from build123d import *

# Parameters (mm, degrees)
SKETCH1_W           = 30
SKETCH1_H           = 38
BOSS_EXTRUDE1_DEPTH = 2
SKETCH2_R           = 0.5
BOSS_EXTRUDE2_DEPTH = 0.8
SKETCH5_W           = 1
SKETCH5_H           = 38
BOSS_EXTRUDE4_DEPTH = 1
SKETCH6_W           = 1
SKETCH6_H           = 38
BOSS_EXTRUDE5_DEPTH = 20
SKETCH8_W           = 18
SKETCH8_H           = 38
BOSS_EXTRUDE6_DEPTH = 3.5
CUT_EXTRUDE1_DEPTH  = 29
SKETCH12_W          = 80
SKETCH12_H          = 38
BOSS_EXTRUDE7_DEPTH = 1


with BuildPart() as part:
    # Sketch1 → Boss-Extrude1 (new body)
    with BuildSketch(Plane.XY):
        Rectangle(SKETCH1_W, SKETCH1_H)
    extrude(amount=BOSS_EXTRUDE1_DEPTH)

    # Sketch2 → Boss-Extrude2 (add)
    with BuildSketch(Plane(origin=(0, 0, 0), x_dir=(-1, 0, 0), z_dir=(0, 0, -1))):
        with Locations(Location((14, 16.5, 0), (0, 0, 180))):
            Circle(SKETCH2_R)
        with Locations(Location((14, -17.5, 0), (0, 0, 180))):
            Circle(SKETCH2_R)
    extrude(amount=BOSS_EXTRUDE2_DEPTH)

    # Sketch5 → Boss-Extrude4 (add)
    with BuildSketch(Plane.XY.offset(2)):
        with Locations((14.5, 0)):
            Rectangle(SKETCH5_W, SKETCH5_H)
    extrude(amount=BOSS_EXTRUDE4_DEPTH)

    # Sketch6 → Boss-Extrude5 (add)
    with BuildSketch(Plane(origin=(15, 0, 0), x_dir=(0, 0, -1), z_dir=(1, 0, 0))):
        with Locations((-2.5, 0)):
            Rectangle(SKETCH6_W, SKETCH6_H)
    extrude(amount=BOSS_EXTRUDE5_DEPTH)

    # Mirror2: part across plane


with BuildPart() as part_1:
    add(part.part)
    add(part.part.mirror(Plane(origin=(25, 0, 0), x_dir=(0, 0, 1), z_dir=(1, 0, 0))))

    # Sketch8 → Boss-Extrude6 (add)
    with BuildSketch(Plane.XY.offset(3)):
        with Locations((25, 0)):
            Rectangle(SKETCH8_W, SKETCH8_H)
    extrude(amount=BOSS_EXTRUDE6_DEPTH)

    # Sketch9 → Cut-Extrude1 (cut)
    with BuildSketch(Plane.ZY.offset(15)):
        Polygon((2, -0.8), (2, 0.8), (1.5, 0.8), (1.5, 1.2), (0.5, 1.2), (0.5, -1.2), (1.5, -1.2), (1.5, -0.8), align=None)
    cut_extrude1 = extrude(amount=-CUT_EXTRUDE1_DEPTH, mode=Mode.SUBTRACT)

    # Mirror3: Cut-Extrude1 across plane
    add(cut_extrude1.mirror(Plane(origin=(25, 0, 0), x_dir=(0, 0, 1), z_dir=(1, 0, 0))), mode=Mode.SUBTRACT)

    # Sketch12 → Boss-Extrude7 (add)
    with BuildSketch(Plane.XY.offset(6.5)):
        with Locations((25, 0)):
            Rectangle(SKETCH12_W, SKETCH12_H)
    extrude(amount=BOSS_EXTRUDE7_DEPTH)


solid = part_1.part
Here's how the part is built. I have some questions about the finished solid (model axes, mm). A direction names the side the tool comes from. Round coordinates to 2 decimals unless told otherwise and drop trailing zeros. Loops run counter-clockwise (first coordinate to the right, second up) from the corner with the lowest first, then second, coordinate; pieces in that order, holes last. Notation, with made-up numbers: (-16, 11) -> (-8, 11) arc R21 cw to (-8, 17) -> close; hole circle Ø5 at (-5.5, -25.75). An arc over 180 degrees is marked (long way). Write each question's results on one line, items separated by ' | '.
(1) If we section it at B-B, the plane y = -6: List the corners of the cut face in (x, z) for me, then the cut area to 3 significant figures.
Worked answers:
outline: (-15, 0) -> (15, 0) -> (15, 2) -> (35, 2) -> (35, 0) -> (65, 0) -> (65, 2) -> (36, 2) -> (36, 3) -> (34, 3) -> (34, 6.5) -> (65, 6.5) -> (65, 7.5) -> (-15, 7.5) -> (-15, 6.5) -> (16, 6.5) -> (16, 3) -> (14, 3) -> (14, 2) -> (-15, 2) -> close | area: 285 mm2
(2) If we section it at A-A, the plane x = 7: List the corners of the cut face in (y, z) for me, then the cut area to 3 significant figures.
Worked answers:
outline: (-19, 0) -> (19, 0) -> (19, 2) -> (0.8, 2) -> (0.8, 1.5) -> (1.2, 1.5) -> (1.2, 0.5) -> (-1.2, 0.5) -> (-1.2, 1.5) -> (-0.8, 1.5) -> (-0.8, 2) -> (-19, 2) -> close; (-19, 6.5) -> (19, 6.5) -> (19, 7.5) -> (-19, 7.5) -> close | area: 111 mm2
(3) For P1, Ø1.5, axis at y = 6.5, z = 3, coming from the -X side; P2, Ø1.5, axis at y = 4.5, z = 5, coming from the -X side; P3, Ø22, axis at x = 23.5, y = 5.5, coming from the -Z side, each with a flat end and sliding along its axis, tell me the tip position at first contact or that it passes through.
Worked answers:
P1: x = 14 | P2: x = 16 | P3: z = 0
(4) If we section it at C-C, the plane z = 3.75: List the corners of the cut face in (x, y) for me.
Worked answers:
outline: (16, -19) -> (34, -19) -> (34, 19) -> (16, 19) -> close
(5) We'd pull the mould along Z, two halves only. Please class faces 5 (the face through (24, 19, 4)), 6 (the face through (16, 0, 5)), 7 (the face through (35, 0, 3)), 8 (the face through (25, 0, 2)): released by +Z, released by -Z, zero draft, split by the parting line, or undercut.
Worked answers:
face 5: zero draft | face 6: undercut | face 7: undercut | face 8: released by -Z
(6) If I drill on L1, parallel to X at y = 13.5, z = 0.5; L2, parallel to Z at x = 60.5, y = -17; L3, parallel to Z at x = 0.5, y = 0.5, over which ranges is the centre line in solid material (lowest first)?
Worked answers:
L1: -15 to 15, 35 to 65 | L2: 0 to 2, 6.5 to 7.5 | L3: 0 to 0.5, 6.5 to 7.5
(7) For faces 1 (the face through (35, 0, 1)), 2 (the face through (-1, 0, 0.5)), 3 (the face through (0, 0, 6.5)), 4 (the face through (51, -10, 2)), which set-ups out of +Z, -Z, +X, -X, +Y, -Y let a thin tool reach every point of the face, with its end or its side?
Worked answers:
face 1: -Z, +Y, -Y | face 2: -X | face 3: -X, +Y, -Y | face 4: +X, +Y, -Y
